Can you work these out from the model? Positions are in its coordinate system, mm. A direction names the side the tool comes from. Give positions to 0.01 mm unless a question says otherwise; leave off trailing zeros. Loops run counter-clockwise (first coordinate to the right, second up) from the corner with the lowest first, then second, coordinate; pieces in that order, holes last. Notation, with made-up numbers: (21.5, 54) - (64.5, 54) arc R5 cw to (64.5, 61) - close; hole circle Ø9 at (-21.5, -7.75). An arc over 180 degrees is marked (long way). Use a Markdown table: item, result. Add a question column.
```python
from build123d import *

# Parameters (mm, degrees)
BOSS_EXTRUDE1_DEPTH = 2.794
FILLET1_R           = 2.54
FILLET2_R           = 12.7
SKETCH2_W           = 2.794
SKETCH2_H           = 6.35
SKETCH2_W_2         = 6.35
SKETCH2_H_2         = 2.794
CUT_EXTRUDE1_DEPTH  = 93.499602356


with BuildPart() as part:
    # Sketch1 → Boss-Extrude1 (new body)
    with BuildSketch(Plane(origin=(0, 0, 0), x_dir=(0, 0, -1), z_dir=(1, 0, 0))):
        Polygon((0, 0), (88.9, 0), (88.9, 12.7), (6.35, 12.7), (6.35, 25.4), (0, 25.4), align=None)
    extrude(amount=BOSS_EXTRUDE1_DEPTH)

    # Fillet1
    fillet1_edges = [part.edges().sort_by_distance(p)[0] for p in [
        (1.397, 25.4, 0),
        (1.397, 25.4, -6.35),
        (1.397, 12.7, -88.9),
        (1.397, 0, -88.9),
    ]]
    fillet(fillet1_edges, radius=FILLET1_R)

    # Fillet2
    fillet2_edges = [part.edges().sort_by_distance(p)[0] for p in [
        (1.397, 0, 0),
    ]]
    fillet(fillet2_edges, radius=FILLET2_R)

    # Sketch2 → Cut-Extrude1 (cut, through all)
    with BuildSketch(Plane.ZY):
        with Locations((-26.797, 3.175)):
            Rectangle(SKETCH2_W, SKETCH2_H)
        with Locations((-81.153, 3.175)):
            Rectangle(SKETCH2_W, SKETCH2_H)
        with Locations((-57.531, 4.953)):
            Rectangle(SKETCH2_W_2, SKETCH2_H_2)
    extrude(amount=-CUT_EXTRUDE1_DEPTH, mode=Mode.SUBTRACT)


solid = part.part
```
1. Suppose I cut it at D-D (y = 5.5). List the corners of the cut face in (x, z) for me, and give its area (3 significant figures).
2. Suppose I cut it at A-A (z = -57.5). List the corners of the cut face in (x, y) for me.
3. Suppose I cut it at B-B (x = 1.25). List the corners of the cut face in (y, z) for me, and give its area (3 significant figures).
4. Suppose I cut it at C-C (y = 1.75). List the corners of the cut face in (x, z) for me.
5. If we mould it in two halves opening along Y, with no side actions, what happens to faces 6 (the face through (1, 3.556, -58)), 7 (the face through (1, 3, -79.756)), 8 (the face through (1, 0, -84))? For each: released by +Y, released by -Y, zero draft, split by the parting line, or undercut.
6. On a 3-axis mill with a long thin cutter (end or side, diameter ignored), from which of +Z, -Z, +X, -X, +Y, -Y can I reach the whole of each face in a straight line? I mean faces 1 (the face through (1.42, 3.62, -3.82)), 2 (the face through (0, 7, -44)), 3 (the face through (1, 6.35, -27)), 4 (the face through (1, 12.7, -47)), 5 (the face through (1, 6.35, -58)). Say none if no direction works.
7. Please list where these lines run through material, in increasing order: line 1 along Z through (x, y) = (0.8, 2.5); line 2 along Z through (x, y) = (2.6, 19.5); line 3 along Y through (x, z) = (1.85, -41.5). Write a range as [from, to].
8. Will these pins go through, and if not, where does the flat tip stop? P1, Ø0.8, axis at x = 2, z = -40, coming from the +Y side; P2, Ø0.8, axis at x = 1.5, y = 3, coming from the +Z side; P3, Ø1.4, axis at x = 2, y = 18.5, coming from the -Z side.
Results below:
| question | item | result |
|---|---|---|
| 1 | outline | (0, -88.9) - (2.79, -88.9) - (2.79, -82.55) - (0, -82.55) - close; (0, -79.76) - (2.79, -79.76) - (2.79, -60.71) - (0, -60.71) - close; (0, -54.36) - (2.79, -54.36) - (2.79, -28.19) - (0, -28.19) - close; (0, -25.4) - (2.79, -25.4) - (2.79, -2.24) - (0, -2.24) - close |
| 1 | area | 209 mm² |
| 2 | outline | (0, 0) - (2.79, 0) - (2.79, 3.56) - (0, 3.56) - close; (0, 6.35) - (2.79, 6.35) - (2.79, 12.7) - (0, 12.7) - close |
| 3 | outline | (0, -86.36) arc R2.54 ccw to (2.54, -88.9) - (10.16, -88.9) arc R2.54 ccw to (12.7, -86.36) - (12.7, -6.35) - (22.86, -6.35) arc R2.54 ccw to (25.4, -3.81) - (25.4, -2.54) arc R2.54 ccw to (22.86, 0) - (12.7, 0) arc R12.7 ccw to (0, -12.7) - (0, -25.4) - (6.35, -25.4) - (6.35, -28.19) - (0, -28.19) - (0, -79.76) - (6.35, -79.76) - (6.35, -82.55) - (0, -82.55) - close; hole (3.56, -60.71) - (6.35, -60.71) - (6.35, -54.36) - (3.56, -54.36) - close |
| 3 | area | 1,120 mm² |
| 4 | outline | (0, -88.77) - (2.79, -88.77) - (2.79, -82.55) - (0, -82.55) - close; (0, -79.76) - (2.79, -79.76) - (2.79, -28.19) - (0, -28.19) - close; (0, -25.4) - (2.79, -25.4) - (2.79, -6.27) - (0, -6.27) - close |
| 5 | face 6 | undercut |
| 5 | face 7 | zero draft |
| 5 | face 8 | released by -Y |
| 6 | face 1 | +Z, +X, -X, -Y |
| 6 | face 2 | +Z, -Z, -X, +Y, -Y |
| 6 | face 3 | +X, -X, -Y |
| 6 | face 4 | -Z, +X, -X, +Y |
| 6 | face 5 | +X, -X |
| 7 | line 1 | [-88.9, -82.55], [-79.76, -28.19], [-25.4, -5.13] |
| 7 | line 2 | [-6.35, 0] |
| 7 | line 3 | [0, 12.7] |
| 8 | P1 | y = 12.7 |
| 8 | P2 | z = -4.05 |
| 8 | P3 | z = -6.35 |
